Build history of the part. All positions in model axes, mm. A direction names the side the tool comes from. Give positions to 0.01 mm unless a question says otherwise; leave off trailing zeros. Loops run counter-clockwise (first coordinate to the right, second up) from the corner with the lowest first, then second, coordinate; pieces in that order, holes last. Notation, with made-up numbers: (83, 32) -> (137, 32) arc R30 ccw to (137, 71) -> close; hole circle Ø8 at (84.25, -19). An arc over 180 degrees is marked (long way). Answer as a JSON object with one key per item and string values. Group by question number.
Q1. Two-plate mould, pull along Z, no slides. Class faces 1 (the flat face through (-33, 0, 0)), 2 (the cylindrical face through (-2.75, -17.58, 0.04)), 3 (the flat face through (-1, 1, -3.175)): pulls with the +Z half, pulls with the -Z half, needs draft (parallel to the pull), parting line crosses it, or undercut.
Q2. Drop flat-ended pins along their axis: pin 1 (1 mm diameter, centred on y = -53.5, z = -0.5, fed in from -X); pin 2 (1 mm diameter, centred on y = -0.5, z = -0.5, fed in from +X). Give the stop position or say it passes through.
Q3. Band-saw the part on A-A, the plane y = 45.5. Write the cut outline in (x, z) (3 decimals), plus the area to 3 significant figures.
Q4. Wall check: probe 1 along Y at (x, z) = (-36, 0); probe 2 along Y at (x, z) = (-4, 2.5); probe 3 along Y at (x, z) = (6.5, 1.75). Give the ranges that are in metal, low to high. Write a range as from..to.
Q5. Tool access for faces 4 (the flat face through (43, -1, 2)), 5 (the flat face through (33, 54, 0)), 6 (the flat face through (-33, 54, 0)): list every direction of +Z, -Z, +X, -X, +Y, -Y with a clear straight run to the whole face (end or side of a thin tool).
Q6. Band-saw the part on C-C, the plane y = 0. Write the cut outline in (x, z) (3 decimals).
Q7. Band-saw the part on B-B, the plane x = 10. Write the cut outline in (y, z) (3 decimals).
from build123d import *

# Parameters (mm, degrees)
SKETCH1_W           = 86
SKETCH1_H           = 131
BOSS_EXTRUDE1_DEPTH = 3.175
SKETCH2_R           = 1.65
CUT_EXTRUDE1_DEPTH  = 10
SKETCH3_R           = 7.5
CUT_EXTRUDE2_DEPTH  = 79.610256964
SKETCH4_R           = 21.1
CUT_EXTRUDE3_DEPTH  = 79.610256964


with BuildPart() as part:
    # Sketch1 → Boss-Extrude1 (new, symmetric)
    with BuildSketch(Plane.XY):
        Rectangle(SKETCH1_W, SKETCH1_H)
    extrude(amount=BOSS_EXTRUDE1_DEPTH, both=True)

    # Sketch2 → Cut-Extrude1 (cut)
    with BuildSketch(Plane.ZY.offset(43)):
        with Locations((0, 54)):
            Circle(SKETCH2_R)
        with Locations((0, -54)):
            Circle(SKETCH2_R)
        Circle(SKETCH2_R)
    cut_extrude1 = extrude(amount=-CUT_EXTRUDE1_DEPTH, mode=Mode.SUBTRACT)

    # Mirror1: Cut-Extrude1 across plane
    add(cut_extrude1.mirror(Plane(origin=(0, 0, 0), x_dir=(0, 0, 1), z_dir=(1, 0, 0))), mode=Mode.SUBTRACT)

    # Sketch3 → Cut-Extrude2 (cut, through all)
    with BuildSketch(Plane.XY.offset(3.175)):
        with Locations((0, 45.5)):
            Circle(SKETCH3_R)
    extrude(amount=-CUT_EXTRUDE2_DEPTH, mode=Mode.SUBTRACT)

    # Sketch4 → Cut-Extrude3 (cut, through all)
    with BuildSketch(Plane.XY.offset(3.175)):
        with Locations((0, -38.5)):
            Circle(SKETCH4_R)
    extrude(amount=-CUT_EXTRUDE3_DEPTH, mode=Mode.SUBTRACT)


solid = part.part
Worked answers:
{
 "1": {"face 1": "undercut", "face 2": "needs draft", "face 3": "pulls with the -Z half"},
 "2": {"pin 1": "x = -33", "pin 2": "x = 33"},
 "3": {"outline": "(-43, -3.175) -> (-7.5, -3.175) -> (-7.5, 3.175) -> (-43, 3.175) -> close; (7.5, -3.175) -> (43, -3.175) -> (43, 3.175) -> (7.5, 3.175) -> close", "area": "451 mm2"},
 "4": {"probe 1": "-65.5..-55.65, -52.35..-1.65, 1.65..52.35, 55.65..65.5", "probe 2": "-65.5..-59.22, -17.78..39.16, 51.84..65.5", "probe 3": "-65.5..-58.57, -18.43..41.76, 49.24..65.5"},
 "5": {"face 4": "+Z, -Z, +X, +Y, -Y", "face 5": "+X", "face 6": "-X"},
 "6": {"outline": "(-43, -3.175) -> (43, -3.175) -> (43, -1.65) -> (33, -1.65) -> (33, 1.65) -> (43, 1.65) -> (43, 3.175) -> (-43, 3.175) -> (-43, 1.65) -> (-33, 1.65) -> (-33, -1.65) -> (-43, -1.65) -> close"},
 "7": {"outline": "(-65.5, -3.175) -> (-57.08, -3.175) -> (-57.08, 3.175) -> (-65.5, 3.175) -> close; (-19.92, -3.175) -> (65.5, -3.175) -> (65.5, 3.175) -> (-19.92, 3.175) -> close"}
}
